Here's how the part is built. I have some questions about the finished solid (model axes, mm). Face numbers are marked on the shaded views. A direction names the side the tool comes from. Coordinates: 2 decimals unless noted, no trailing zeros. Write each loop counter-clockwise with the first axis right and the second up, starting at its lowest first coordinate (ties: lowest second). Pieces come first, ordered by that corner, then holes.
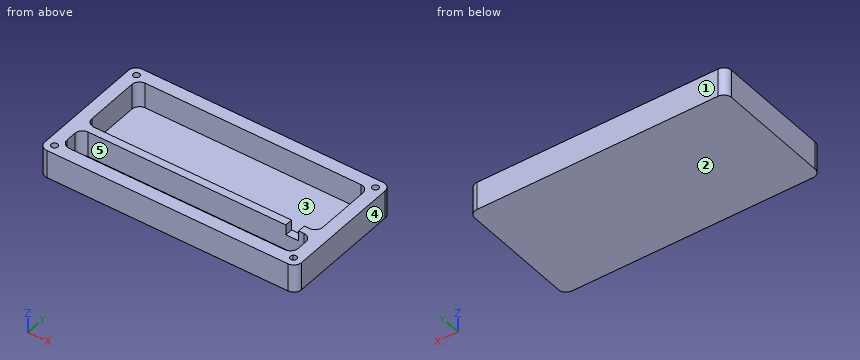
```python
from build123d import *

# Parameters (mm, degrees)
F0_W      = 100
F0_H      = 50
F1_DEPTH  = 1
F2_W      = 100
F2_H      = 50
F2_W_2    = 90
F2_H_2    = 40
F3_DEPTH  = 10
F4_W      = 90
F4_H      = 3
F5_DEPTH  = 11
F6_W      = 5
F6_H      = 4
F7_DEPTH  = 3
F8_R      = 3
F9_R      = 1.25
F10_DEPTH = 6


with BuildPart() as f1:
    # F0 (on Top) → F1 (new body)
    with BuildSketch(Plane.XY):
        Rectangle(F0_W, F0_H)
    extrude(amount=F1_DEPTH)

    # F2 (on face) → F3 (join)
    with BuildSketch(Plane.XY.offset(1)):
        Rectangle(F2_W, F2_H)
        Rectangle(F2_W_2, F2_H_2, mode=Mode.SUBTRACT)
    extrude(amount=F3_DEPTH)

    # F4 (on Top) → F5 (join, through all)
    with BuildSketch(Plane.XY):
        with Locations((0, -8.5)):
            Rectangle(F4_W, F4_H)
    extrude(amount=F5_DEPTH)

    # F6 (on face) → F7 (cut, through all)
    with BuildSketch(Plane(origin=(0, -7, 0), x_dir=(-1, 0, 0), z_dir=(0, 1, 0))):
        with Locations((-37.5, 9)):
            Rectangle(F6_W, F6_H)
    extrude(amount=-F7_DEPTH, mode=Mode.SUBTRACT)

    # F8
    f8_edges = [f1.edges().sort_by_distance(p)[0] for p in [
        (50, -25, 5.5),
        (50, 25, 5.5),
        (-50, -25, 5.5),
        (-50, 25, 5.5),
        (45, -20, 6),
        (-45, -20, 6),
        (45, 20, 6),
        (-45, 20, 6),
        (45, -7, 6),
        (-45, -7, 6),
        (45, -10, 6),
        (-45, -10, 6),
    ]]
    fillet(f8_edges, radius=F8_R)

    # F9 (on face) → F10 (cut)
    with BuildSketch(Plane.XY.offset(11)):
        with BuildLine():
            ThreePointArc((46.556349, -22.806349), (47.440233, -22.440233), (47.806349, -21.556349))
            ThreePointArc((47.806349, -21.556349), (47.034703, -20.4015), (45.672466, -20.672466))
            Line((45.672466, -20.672466), (46.556349, -21.556349))
            Line((46.556349, -21.556349), (46.556349, -22.806349))
        make_face()
        with BuildLine():
            Line((46.556349, -21.556349), (45.672466, -20.672466))
            ThreePointArc((45.672466, -20.672466), (45.4015, -22.034703), (46.556349, -22.806349))
            Line((46.556349, -22.806349), (46.556349, -21.556349))
        make_face()
        with Locations((-46.556349, -21.556349)):
            Circle(F9_R)
        with Locations((-46.556349, 21.556349)):
            Circle(F9_R)
        with Locations((46.556349, 21.556349)):
            Circle(F9_R)
    extrude(amount=-F10_DEPTH, mode=Mode.SUBTRACT)


solid = f1.part
```
1) Imagine slicing it at B-B on x = 32. Please give me the cut outline in (y, z).
Values follow:
outline: (-25, 0) - (25, 0) - (25, 11) - (20, 11) - (20, 1) - (-7, 1) - (-7, 11) - (-10, 11) - (-10, 1) - (-20, 1) - (-20, 11) - (-25, 11) - close
2) Will these pins go through, and if not, where does the flat tip stop? pin 1 (13.5 mm diameter, centred on x = 12.5, y = 0, fed in from +Z); pin 2 (0.8 mm diameter, centred on x = -46.5, y = 21, fed in from +Z); pin 3 (0.9 mm diameter, centred on x = 37.5, y = -8.5, fed in from +Z).
Values follow:
pin 1: stops at z = 1
pin 2: stops at z = 5
pin 3: stops at z = 7
3) Imagine slicing it at A-A on z = 2.5. Please give me the cut outline in (x, y), then the cut area to 3 significant figures.
Values follow:
outline: (-50, -22) arc R3 ccw to (-47, -25) - (47, -25) arc R3 ccw to (50, -22) - (50, 22) arc R3 ccw to (47, 25) - (-47, 25) arc R3 ccw to (-50, 22) - close; hole (-45, -17) arc R3 ccw to (-42, -20) - (42, -20) arc R3 ccw to (45, -17) - (45, -13) arc R3 ccw to (42, -10) - (-42, -10) arc R3 ccw to (-45, -13) - close; hole (-45, -4) arc R3 ccw to (-42, -7) - (42, -7) arc R3 ccw to (45, -4) - (45, 17) arc R3 ccw to (42, 20) - (-42, 20) arc R3 ccw to (-45, 17) - close
area: 1,680 mm2
4) On a 3-axis mill with a long thin cutter (end or side, diameter ignored), from which of +Z, -Z, +X, -X, +Y, -Y can I reach the whole of each face in a straight line? I mean the marked faces 4 and 5. Say none if no direction works.
Values follow:
face 4: +Z, -Z, +X, +Y, -Y
face 5: +Z
5) Imagine slicing it at C-C on y = -15.5. Please give me the cut outline in (x, z).
Values follow:
outline: (-50, 0) - (50, 0) - (50, 11) - (45, 11) - (45, 1) - (-45, 1) - (-45, 11) - (-50, 11) - close
6) I need wall thicknesses on probe 1 along Y at (x, z) = (19, 3); probe 2 along X at (y, z) = (7.5, 4.5); probe 3 along X at (y, z) = (-5.5, 10.25). Which ranges of each line are inside material? Lowest first, please.
Values follow:
probe 1: y = -25 to -20, -10 to -7, 20 to 25
probe 2: x = -50 to -45, 45 to 50
probe 3: x = -50 to -44.6, 44.6 to 50
7) We'd pull the mould along Y, two halves only. Please class the marked faces 1, 2 and 3: pulls with the +Y half, pulls with the -Y half, needs draft (parallel to the pull), parting line crosses it, or undercut.
Values follow:
face 1: pulls with the +Y half
face 2: needs draft
face 3: undercut
